```python
from build123d import *

# Parameters (mm, degrees)
MODEL_R                 = 1.5
SALIENTE_EXTRUIR1_DEPTH = 3


with BuildPart() as part:
    # Model → Saliente-Extruir1 (new body)
    with BuildSketch(Plane.XY):
        with BuildLine():
            Line((152.34213351, 211.823953209), (158.34213351, 211.823953209))
            ThreePointArc((158.34213351, 211.823953209), (161.524114025, 210.505933724), (162.84213351, 207.323953209))
            Line((162.84213351, 207.323953209), (162.84213351, 198.323953209))
            ThreePointArc((162.84213351, 198.323953209), (158.34213351, 193.823953209), (153.84213351, 198.323953209))
            Line((153.84213351, 198.323953209), (153.84213351, 202.823953209))
            Line((153.84213351, 202.823953209), (152.34213351, 202.823953209))
            ThreePointArc((152.34213351, 202.823953209), (147.84213351, 207.323953209), (152.34213351, 211.823953209))
        make_face()
        with Locations((158.34213351, 207.323953209)):
            Circle(MODEL_R, mode=Mode.SUBTRACT)
        with Locations((158.34213351, 198.323953209)):
            Circle(MODEL_R, mode=Mode.SUBTRACT)
    extrude(amount=SALIENTE_EXTRUIR1_DEPTH)


solid = part.part
```
The model under review builds one solid part; all positions refer to its coordinate system, in mm. A direction names the side the tool comes from. Coordinates: 2 decimals unless noted, no trailing zeros. Write each loop counter-clockwise with the first axis right and the second up, starting at its lowest first coordinate (ties: lowest second). Pieces come first, ordered by that corner, then holes.
1) The part is to be moulded in two halves that separate along Y. For faces 3 (the face through (158.441, 193.825, 1.479)), 4 (the face through (155, 211.824, 1)), 5 (the face through (157.152, 197.411, 1.479)), say which applies: pulls with the +Y half, pulls with the -Y half, needs draft (parallel to the pull), parting line crosses it, or undercut.
2) To check wall thickness, follow probe 1 along Y at (x, z) = (153.75, 2.85); probe 2 along X at (y, z) = (202, 1.8); probe 3 along Y at (x, z) = (159.25, 2.6). State the ranges of each line that lie inside material, in increasing order.
3) We need section C-C on x = 159. State the section outline as (y, z) points, then the cut area to 3 significant figures.
4) We need section D-D on y = 207.75. State the section outline as (x, z) points, then the cut area to 3 significant figures.
5) Machinability: for faces 1 (the face through (153, 202.824, 1)), 2 (the face through (157, 205, 0)), which of the approach directions +Z, -Z, +X, -X, +Y, -Y give a long, thin tool a straight path to every point of the face, cutting with its end or side? Answer none if there is none.
6) We need section A-A on z = 0.8. State the section outline as (x, y) points.
7) We need section B-B on y = 197.25. State the section outline as (x, z) points.
8) Clearance check with a flat-ended pin moving along its axis: pin 1 Ø1.5 at (y, z) = (199.5, 0.5) entering from -X. State where the tip first meets the part, or that it passes through.
Answer list:
1. face 3: pulls with the -Y half
1. face 4: pulls with the +Y half
1. face 5: undercut
2. probe 1: y = 202.82 to 211.82
2. probe 2: x = 153.84 to 162.84
2. probe 3: y = 193.92 to 197.13, 199.52 to 206.13, 208.52 to 211.73
3. outline: (193.87, 0) - (196.98, 0) - (196.98, 3) - (193.87, 3) - close; (199.67, 0) - (205.98, 0) - (205.98, 3) - (199.67, 3) - close; (208.67, 0) - (211.78, 0) - (211.78, 3) - (208.67, 3) - close
3. area: 37.5 mm2
4. outline: (147.86, 0) - (156.9, 0) - (156.9, 3) - (147.86, 3) - close; (159.78, 0) - (162.82, 0) - (162.82, 3) - (159.78, 3) - close
4. area: 36.2 mm2
5. face 1: +Z, -Z, -X, -Y
5. face 2: -Z, +X, -X, +Y, -Y
6. outline: (152.34, 202.82) - (153.84, 202.82) - (153.84, 198.32) arc R4.5 ccw to (162.84, 198.32) - (162.84, 207.32) arc R4.5 ccw to (158.34, 211.82) - (152.34, 211.82) arc R4.5 ccw to start; hole circle Ø3 at (158.34, 198.32); hole circle Ø3 at (158.34, 207.32)
7. outline: (153.97, 0) - (157.29, 0) - (157.29, 3) - (153.97, 3) - close; (159.39, 0) - (162.71, 0) - (162.71, 3) - (159.39, 3) - close
8. pin 1: stops at x = 153.84
